```python
from build123d import *

# Parameters (mm, degrees)
SKETCH1_W           = 160
SKETCH1_H           = 160
BOSS_EXTRUDE1_DEPTH = 9
SKETCH2_W           = 9
SKETCH2_H           = 15
SKETCH2_H_2         = 9
BOSS_EXTRUDE2_DEPTH = 9
SKETCH3_R           = 1.7
SKETCH3_W           = 9
SKETCH3_H           = 15
CUT_EXTRUDE1_DEPTH  = 121.008333044
CUT_EXTRUDE2_DEPTH  = 121.008333044
SKETCH5_R           = 9.5
SKETCH5_R_2         = 2.75
CUT_EXTRUDE3_DEPTH  = 121.008333044
SKETCH6_W           = 160
SKETCH6_H           = 9
BOSS_EXTRUDE3_DEPTH = 1
SKETCH7_R           = 11.8
CUT_EXTRUDE4_DEPTH  = 121.008333044
SKETCH8_R           = 14.825
CUT_EXTRUDE5_DEPTH  = 264.594385373


with BuildPart() as part:
    # Sketch1 → Boss-Extrude1 (new body)
    with BuildSketch(Plane(origin=(0, 0, 0), x_dir=(1, 0, 0), z_dir=(0, 1, 0))):
        Rectangle(SKETCH1_W, SKETCH1_H)
    boss_extrude1 = extrude(amount=BOSS_EXTRUDE1_DEPTH)

    # Sketch2 → Boss-Extrude2 (add)
    with BuildSketch(Plane(origin=(0, 9, 0), x_dir=(1, 0, 0), z_dir=(0, 1, 0))):
        with Locations((-84.5, 0)):
            Rectangle(SKETCH2_W, SKETCH2_H)
        with Locations((-84.5, 43.75)):
            Rectangle(SKETCH2_W, SKETCH2_H)
        with Locations((-84.5, -43.75)):
            Rectangle(SKETCH2_W, SKETCH2_H)
        with Locations((-84.5, 75.5)):
            Rectangle(SKETCH2_W, SKETCH2_H_2)
        with Locations((-84.5, -75.5)):
            Rectangle(SKETCH2_W, SKETCH2_H_2)
    boss_extrude2 = extrude(amount=-BOSS_EXTRUDE2_DEPTH)

    # Sketch3 → Cut-Extrude1 (cut, through all)
    with BuildSketch(Plane(origin=(0, 9, 0), x_dir=(1, 0, 0), z_dir=(0, 1, 0))):
        with Locations(Location((70.5, 21.875, 0), (0, 0, 270))):
            Circle(SKETCH3_R)
        with Locations(Location((70.5, -21.875, 0), (0, 0, 270))):
            Circle(SKETCH3_R)
        with Locations((70.5, 43.75)):
            Rectangle(SKETCH3_W, SKETCH3_H)
        with Locations((70.5, 0)):
            Rectangle(SKETCH3_W, SKETCH3_H)
        with Locations((70.5, -43.75)):
            Rectangle(SKETCH3_W, SKETCH3_H)
    cut_extrude1 = extrude(amount=-CUT_EXTRUDE1_DEPTH, mode=Mode.SUBTRACT)

    # Sketch4 → Cut-Extrude2 (cut, through all)
    with BuildSketch(Plane(origin=(0, 9, 0), x_dir=(1, 0, 0), z_dir=(0, 1, 0))):
        Polygon((-80, 23.575), (-76.2, 23.575), (-76.2, 24.625), (-74, 24.625), (-74, 23.575), (-71, 23.575), (-71, 20.175), (-74, 20.175), (-74, 19.125), (-76.2, 19.125), (-76.2, 20.175), (-80, 20.175), align=None)
        Polygon((-80, -23.575), (-80, -20.175), (-76.2, -20.175), (-76.2, -19.125), (-74, -19.125), (-74, -20.175), (-71, -20.175), (-71, -23.575), (-74, -23.575), (-74, -24.625), (-76.2, -24.625), (-76.2, -23.575), align=None)
    cut_extrude2 = extrude(amount=-CUT_EXTRUDE2_DEPTH, mode=Mode.SUBTRACT)

    # Sketch5 → Cut-Extrude3 (cut, through all)
    with BuildSketch(Plane(origin=(0, 9, 0), x_dir=(1, 0, 0), z_dir=(0, 1, 0))):
        with Locations(Location((0, 0, 0), (0, 0, 270))):
            Circle(SKETCH5_R)
        with Locations(Location((-20, 40.25, 0), (0, 0, 270))):
            Circle(SKETCH5_R_2)
        with Locations(Location((20, 40.25, 0), (0, 0, 270))):
            Circle(SKETCH5_R_2)
        with Locations(Location((20, -40.25, 0), (0, 0, 270))):
            Circle(SKETCH5_R_2)
        with Locations(Location((-20, -40.25, 0), (0, 0, 270))):
            Circle(SKETCH5_R_2)
    extrude(amount=-CUT_EXTRUDE3_DEPTH, mode=Mode.SUBTRACT)

    # Sketch6 → Boss-Extrude3 (add)
    with BuildSketch(Plane(origin=(80, 0, 0), x_dir=(0, 0, -1), z_dir=(1, 0, 0))):
        with Locations((0, 4.5)):
            Rectangle(SKETCH6_W, SKETCH6_H)
    boss_extrude3 = extrude(amount=BOSS_EXTRUDE3_DEPTH)

    # Sketch7 → Cut-Extrude4 (cut, through all)
    with BuildSketch(Plane(origin=(0, 9, 0), x_dir=(1, 0, 0), z_dir=(0, 1, 0))):
        with Locations(Location((41, 50, 0), (0, 0, 270))):
            Circle(SKETCH7_R)
    cut_extrude4 = extrude(amount=-CUT_EXTRUDE4_DEPTH, mode=Mode.SUBTRACT)

    # Mirror1: Boss-Extrude1, Boss-Extrude2, Cut-Extrude1, Cut-Extrude2, Boss-Extrude3, Cut-Extrude4 across plane
    add(boss_extrude1.mirror(Plane.ZY.offset(-81)))
    add(boss_extrude2.mirror(Plane.ZY.offset(-81)))
    add(cut_extrude1.mirror(Plane.ZY.offset(-81)), mode=Mode.SUBTRACT)
    add(cut_extrude2.mirror(Plane.ZY.offset(-81)), mode=Mode.SUBTRACT)
    add(boss_extrude3.mirror(Plane.ZY.offset(-81)))
    add(cut_extrude4.mirror(Plane.ZY.offset(-81)), mode=Mode.SUBTRACT)

    # Sketch8 → Cut-Extrude5 (cut, through all)
    with BuildSketch(Plane(origin=(0, 9, 0), x_dir=(1, 0, 0), z_dir=(0, 1, 0))):
        with Locations(Location((135.462999704, 0, 0), (0, 0, 270))):
            Circle(SKETCH8_R)
        with Locations(Location((187.146093847, 18.811107883, 0), (0, 0, 270))):
            Circle(SKETCH8_R)
        with Locations(Location((202.537000296, -23.475060052, 0), (0, 0, 270))):
            Circle(SKETCH8_R)
        with Locations(Location((150.853906153, -42.286167935, 0), (0, 0, 270))):
            Circle(SKETCH8_R)
    extrude(amount=-CUT_EXTRUDE5_DEPTH, mode=Mode.SUBTRACT)


solid = part.part
```
Part model, mm, in its own coordinate system. A direction names the side the tool comes from. Give positions to 0.01 mm unless a question says otherwise; leave off trailing zeros. Write each loop counter-clockwise with the first axis right and the second up, starting at its lowest first coordinate (ties: lowest second). Pieces come first, ordered by that corner, then holes. Notation, with made-up numbers: (68.5, 55) -> (122.5, 55) arc R27 ccw to (122.5, 75) -> close; hole circle Ø3 at (-11, 11.5). An arc over 180 degrees is marked (long way). Put each result on its own line as item: value. Start each with the question number.
Item 1: Wall check: L1, parallel to X at y = 7.25, z = 0; L2, parallel to Z at x = 235, y = 6.5 (3 decimals); L3, parallel to Z at x = 203.5, y = 3.25. Give the ranges that are in metal, low to high. Write a range as [from, to].
Item 2: Pull direction Z, two halves, no side cores. Call faces 6 (the face through (-80, 4, 61)), 7 (the face through (83, 4, 80)), 8 (the face through (-89, 5, 44)): pulls with the +Z half, pulls with the -Z half, needs draft (parallel to the pull), parting line crosses it, or undercut.
Item 3: Which spindle directions (+Z, -Z, +X, -X, +Y, -Y) get a long thin tool onto all of the face, cutting with end or side? Do faces 1 (the face through (66, 5, 0)), 2 (the face through (-89, 5, -75)), 3 (the face through (251, 5, 0)), 4 (the face through (242, 4, 30)), 5 (the face through (-80, 4, -61)). Say none if no direction does.
Item 4: Cut at C-C (y = 3.75). State how many separate pieces and enclosed holes the cut face has, then the cut area to 3 significant figures.
Item 5: Pin check, flat tips, straight feed: pin 1 Ø1 at (y, z) = (6, -21.5) entering from +X; pin 2 Ø1.5 at (y, z) = (8, 52.5) entering from -X; pin 3 Ø2 at (y, z) = (2, -16.5) entering from +X. Stop position of each tip, or through.
Item 6: Cut at B-B (x = 126). List the corners of the cut face in (y, z).
Item 7: Cut at A-A (z = 0). List the corners of the cut face in (x, y), then the cut area to 3 significant figures.
Answer list:
1. L1: x = [-89, -9.5], [9.5, 66], [75, 87], [96, 120.64], [150.29, 251]
1. L2: z = [-80, -23.575], [-20.175, 20.175], [23.575, 80]
1. L3: z = [-80, 8.68], [38.27, 80]
2. face 6: undercut
2. face 7: pulls with the +Z half
2. face 8: needs draft
3. face 1: +Y, -Y
3. face 2: +Z, -Z, -X, +Y, -Y
3. face 3: +Z, -Z, +X, +Y, -Y
3. face 4: +X, +Y, -Y
3. face 5: -X, +Y, -Y
4. separate pieces: 1
4. enclosed holes: 21
4. area: 47,700 mm2
5. pin 1: stops at x = 233
5. pin 2: stops at x = -80
5. pin 3: stops at x = 242
6. outline: (0, -80) -> (9, -80) -> (9, -60.69) -> (0, -60.69) -> close; (0, -39.31) -> (9, -39.31) -> (9, -11.41) -> (0, -11.41) -> close; (0, 11.41) -> (9, 11.41) -> (9, 80) -> (0, 80) -> close
7. outline: (-89, 0) -> (-9.5, 0) -> (-9.5, 9) -> (-89, 9) -> close; (9.5, 0) -> (66, 0) -> (66, 9) -> (9.5, 9) -> close; (75, 0) -> (87, 0) -> (87, 9) -> (75, 9) -> close; (96, 0) -> (120.64, 0) -> (120.64, 9) -> (96, 9) -> close; (150.29, 0) -> (251, 0) -> (251, 9) -> (150.29, 9) -> close
7. area: 2,460 mm2
